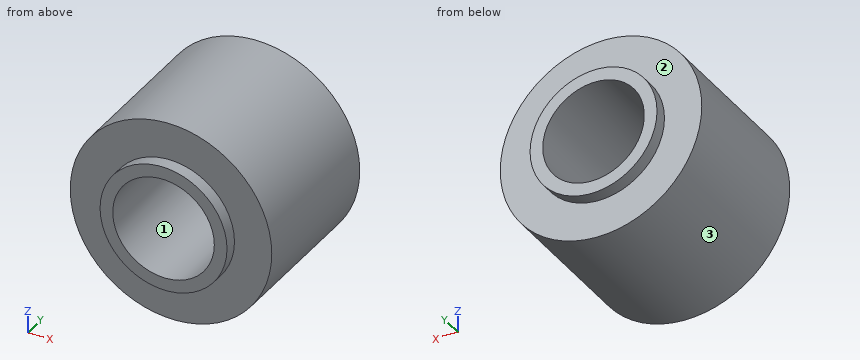
```python
from build123d import *

# Parameters (mm, degrees)
SKETCH1_W = 3.1496
SKETCH1_H = 11.1125
SKETCH2_W = 2.35
SKETCH2_H = 0.80625


with BuildPart() as part:
    # Sketch1 → Revolve1 (revolve)
    with BuildSketch(Plane.XY):
        with Locations((4.7752, 0)):
            Rectangle(SKETCH1_W, SKETCH1_H)
    revolve(axis=Axis((0, 5.55625, 0), (0, -1, 0)))

    # Sketch2 → Cut-Revolve1 (revolve, cut)
    with BuildSketch(Plane.XY):
        with Locations((-5.175, 5.153125)):
            Rectangle(SKETCH2_W, SKETCH2_H)
        with Locations((-5.175, -5.153125)):
            Rectangle(SKETCH2_W, SKETCH2_H)
    revolve(axis=Axis((0, -6.044864414, 0), (0, 1, 0)), mode=Mode.SUBTRACT)


solid = part.part
```
Check sheet for the modelled part. Datum: model origin and axes. Units: mm. Face numbers are marked on the shaded views. Round coordinates to 2 decimals unless told otherwise and drop trailing zeros. Loops run counter-clockwise (first coordinate to the right, second up) from the corner with the lowest first, then second, coordinate; pieces in that order, holes last. Notation, with made-up numbers: (42.5, -24) - (71.5, -24) arc R9 ccw to (71.5, -14) - close; hole circle Ø1 at (6.5, 4). An arc over 180 degrees is marked (long way). Answer as a JSON object with one key per item and string values. Group by question number.
Q1. Sectioned sample at B-B, the plane x = 0. Enter the section's corners in (y, z), plus the area to 3 significant figures.
Q2. Sectioned sample at C-C, the plane y = -4.5. Enter the section's corners in (x, z).
Q3. Sectioned sample at A-A, the plane z = 0. Enter the section's corners in (x, y), plus the area to 3 significant figures.
Q4. Scan lines: line 1 along Z through (x, y) = (0, 1.5); line 2 along Y through (x, z) = (3, 3.5); line 3 along X through (y, z) = (-3, -0.75). Record each from-to range of solid material in increasing order. Write a range as [from, to].
Q5. Gauge pin test, flat ends, axial feed: P1, Ø5, axis at y = -2.5, z = 3, coming from the +X side; P2, Ø6.5, axis at x = -1, z = -2, coming from the +Y side; P3, Ø1, axis at y = -3.5, z = -4, coming from the +X side. Record the tip position at first contact, or that the pin passes through.
Q6. Sectioned sample at D-D, the plane x = -5. Enter the section's corners in (y, z), plus the area to 3 significant figures.
Q7. Mould release check, pull along X, two halves, no side actions. Record for the marked faces 1, 2 and 3: released by +X, released by -X, zero draft, split by the parting line, or undercut.
Solution:
{
 "1": {"outline": "(-5.56, -4) - (-4.75, -4) - (-4.75, -6.35) - (4.75, -6.35) - (4.75, -4) - (5.56, -4) - (5.56, -3.2) - (-5.56, -3.2) - close; (-5.56, 3.2) - (5.56, 3.2) - (5.56, 4) - (4.75, 4) - (4.75, 6.35) - (-4.75, 6.35) - (-4.75, 4) - (-5.56, 4) - close", "area": "62.4 mm²"},
 "2": {"outline": "circle Ø12.7 at (0, 0); hole circle Ø6.4 at (0, 0)"},
 "3": {"outline": "(-6.35, -4.75) - (-4, -4.75) - (-4, -5.56) - (-3.2, -5.56) - (-3.2, 5.56) - (-4, 5.56) - (-4, 4.75) - (-6.35, 4.75) - close; (3.2, -5.56) - (4, -5.56) - (4, -4.75) - (6.35, -4.75) - (6.35, 4.75) - (4, 4.75) - (4, 5.56) - (3.2, 5.56) - close", "area": "62.4 mm²"},
 "4": {"line 1": "z = [-6.35, -3.2], [3.2, 6.35]", "line 2": "y = [-4.75, 4.75]", "line 3": "x = [-6.31, -3.11], [3.11, 6.31]"},
 "5": {"P1": "stops at x = 6.33", "P2": "stops at y = 5.56", "P3": "stops at x = 5.3"},
 "6": {"outline": "(-4.75, -3.91) - (4.75, -3.91) - (4.75, 3.91) - (-4.75, 3.91) - close", "area": "74.4 mm²"},
 "7": {"face 1": "undercut", "face 2": "zero draft", "face 3": "split by the parting line"}
}
